Autodesk Inventor part; units mm, degrees
ref_plane "YZ Plane" through (0, 0, 0) normal (1, 0, 0) x (0, 1, 0)
ref_plane "XZ Plane" through (0, 0, 0) normal (0, 1, 0) x (-1, 0, 0)
ref_plane "XY Plane" through (0, 0, 0) normal (0, 0, 1) x (1, 0, 0)
sketch "Sketch1" plane through (0, 0, 0) normal (0, 0, 1) x (1, 0, 0)
  line L0 (-3.125, -3.125) -> (3.125, -3.125)
  line L1 (3.125, -3.125) -> (3.125, 3.125)
  line L2 (3.125, 3.125) -> (-3.125, 3.125)
  line L3 (-3.125, 3.125) -> (-3.125, -3.125)
  line L4 (-3.125, -3.125) -> (3.125, 3.125) construction
  line L5 (3.125, -3.125) -> (-3.125, 3.125) construction
  point P0 (0, 0)
  dimension "d0" = 6.25
  dimension "d1" = 6.25
extrude "Extrusion1" add sketch "Sketch1" along normal mid plane 6.25
sketch "Sketch2" plane through (0, 0, 0) normal (1, 0, 0) x (0, 1, 0)
  line L0 (-3.125, 3.125) -> (3.125, 3.125)
  line L1 (2, 4.375) -> (2, 8.375)
  line L2 (2, 8.375) -> (2.25, 8.375)
  line L3 (2.25, 8.375) -> (1.625, 11.875)
  line L4 (0, 0) -> (0, 14.1963) construction
  line L5 (1.625, 11.875) -> (1.625, 13.125)
  line L6 (2, 4.375) -> (2.5, 3.125)
  line L7 (1.25, 13.125) -> (1.25, 11.8418)
  line L8 (1.25, 11.8418) -> (1.8021, 8.75)
  line L9 (1.8021, 8.75) -> (1.625, 8.75)
  line L10 (1.625, 8.75) -> (1.625, 4.3028)
  line L11 (1.625, 4.3028) -> (2.1518, 2.9857)
  line L12 (1.625, 13.125) -> (1.25, 13.125)
  point P0 (2.0961, 3.125)
  dimension "d4" = 4
  dimension "d5" = 4.5
  dimension "d6" = 3.25
  dimension "d7" = 10
  dimension "d8" = 1.25
  dimension "d9" = 3.5
  dimension "d11" = 5
  dimension "d12" = 1.25
  dimension "d13" = 2.5
revolve "Revolution1" add sketch "Sketch2" angle 360 about axis through (0, 0, 0) along (0, 0, 1)
pattern_circular "Circular Pattern1" count 3 over 180 about axis through (0, -10, 0) along (0, 1, 0) of "Revolution1"
equation "\"d2\" = d1"
properties part number "Adafruit_4662"
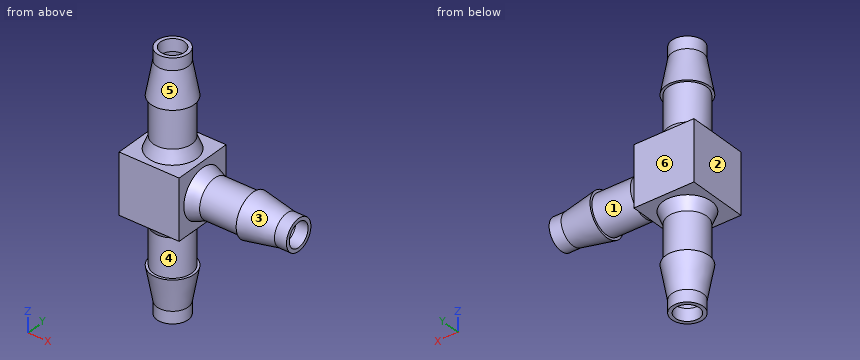
Here's how the part is built. I have some questions about the finished solid (model axes, mm). Face numbers are marked on the shaded views. A direction names the side the tool comes from. Round coordinates to 2 decimals unless told otherwise and drop trailing zeros. Order: outer loops, then holes, each group sorted by start corner. A loop starts at its lowest first (then second) coordinate and runs counter-clockwise, first axis right, second up. Notation, with made-up numbers: M -27.5,-7.5 L 25.5,-7.5 A23 cw 25.5,12.5 Z; hole C -17,73 d8. An arc over 180 degrees is marked long. Use CSV: the item, a comma, the result in double quotes.
1) I want a section at A-A (z = 0). List the corners of the cut face in (x, y) for me (3 decimals).
Taken from the geometry:
outline,"M -3.125,-3.125 L 3.125,-3.125 L 3.125,-2.5 L 4.375,-2 L 8.375,-2 L 8.375,-2.25 L 11.875,-1.625 L 13.125,-1.625 L 13.125,-1.25 L 11.842,-1.25 L 8.75,-1.802 L 8.75,-1.625 L 4.303,-1.625 L 3.125,-2.096 L 3.125,2.096 L 4.303,1.625 L 8.75,1.625 L 8.75,1.802 L 11.842,1.25 L 13.125,1.25 L 13.125,1.625 L 11.875,1.625 L 8.375,2.25 L 8.375,2 L 4.375,2 L 3.125,2.5 L 3.125,3.125 L -3.125,3.125 Z"
2) On a 3-axis mill with a long thin cutter (end or side, diameter ignored), from which of +Z, -Z, +X, -X, +Y, -Y can I reach the whole of each face in a straight line? I mean the marked faces 1 and 2. Say none if no direction works.
Taken from the geometry:
face 1,"none"
face 2,"+Z, -Z, -X, +Y, -Y"
3) I'm going to push flat-ended pins straight in: P1, Ø1, axis at x = 4, y = 1.5, coming from the -Z side; P2, Ø3, axis at x = 11, z = 4, coming from the -Y side; P3, Ø2, axis at x = 0, y = 0, coming from the +Z side (3 decimals); P4, Ø2, axis at x = 9, y = -1.5, coming from the -Z side. Where does each tip first touch, or does it pass through?
Taken from the geometry:
P1,"z = -1.99"
P2,"through"
P3,"z = 3.125"
P4,"z = -2.14"
4) If we mould it in two halves opening along Z, with no side actions, what happens to the marked faces 3, 4, 5 and 6? For each: pulls with the +Z half, pulls with the -Z half, needs draft (parallel to the pull), parting line crosses it, or undercut.
Taken from the geometry:
face 3,"parting line crosses it"
face 4,"undercut"
face 5,"pulls with the +Z half"
face 6,"needs draft"
5) I need wall thicknesses on line 1 along X through (y, z) = (0, 5.85) (3 decimals); line 2 along Y through (x, z) = (0, 12.85) (3 decimals). Which ranges of each line are inside material? Lowest first, please. Write a range as [from, to].
Taken from the geometry:
line 1,"[-2, -1.625], [1.625, 2]"
line 2,"[-1.625, -1.25], [1.25, 1.625]"
6) I want a section at B-B (x = 6). List the corners of the cut face in (y, z) for me (3 decimals), then the cut area to 3 significant figures.
Taken from the geometry:
outline,"C 0,0 d4; hole C 0,0 d3.25"
area,"4.27 mm^2"
